Build history of the part. All positions in model axes, mm. A direction names the side the tool comes from. Coordinates: 2 decimals unless noted, no trailing zeros. Order: outer loops, then holes, each group sorted by start corner. A loop starts at its lowest first (then second) coordinate and runs counter-clockwise, first axis right, second up. Notation, with made-up numbers: M 13,-3 L 20,-3 A26 ccw 20,31 Z; hole C 15,63.5 d1. An arc over 180 degrees is marked long. Write item = value, one per line. Start each with the question number.
Q1. Pin check, flat tips, straight feed: P1, Ø3, axis at y = 0, z = 0.5, coming from the +X side; P2, Ø4, axis at y = 0, z = 0, coming from the -X side. Stop position of each tip, or through.
Q2. Drill centre lines: probe 1 along Y at (x, z) = (-0.85, 0); probe 2 along X at (y, z) = (2.25, -3). Where is each one in solid material? Low to high.
Q3. Band-saw the part on D-D on z = -4. Write the cut outline in (x, y).
Q4. Band-saw the part on C-C on x = -1.1. Write the cut outline in (y, z), plus the area to 3 significant figures.
Q5. 3-axis set-ups, long thin cutter, end or side, ignore diameter. For faces 4 (the face through (-1.51, -1.08, 4.88)), 5 (the face through (-0.5, 3.3, -0.1)): which of +Z, -Z, +X, -X, +Y, -Y reach the whole face in a straight line?
Q6. Band-saw the part on A-A on z = 0. Write the cut outline in (x, y).
Q7. Pull direction Z, two halves, no side cores. Call faces 1 (the face through (-0.3, -3, -0.1)), 2 (the face through (0, 2, 1)), 3 (the face through (-1.237, 1.617, -0.67)): released by +Z, released by -Z, zero draft, split by the parting line, or undercut.
Autodesk Inventor part; units mm, degrees
ref_plane "YZ Plane" through (0, 0, 0) normal (1, 0, 0) x (0, 1, 0)
ref_plane "XZ Plane" through (0, 0, 0) normal (0, 1, 0) x (-1, 0, 0)
ref_plane "XY Plane" through (0, 0, 0) normal (0, 0, 1) x (1, 0, 0)
sketch "Эскиз1" plane through (0, 0, 0) normal (0, 0, 1) x (1, 0, 0)
  line L0 (0, 1.75) -> (0, 3)
  line L1 (0, 3) -> (-0.5, 3)
  line L2 (-0.5, 3) -> (-0.5, 5)
  line L3 (-0.5, 5) -> (-2.5, 5)
  line L4 (-2.5, 5) -> (-2.5, 1.75)
  line L5 (-2.5, 1.75) -> (0, 1.75)
  line L6 (0, 0) -> (-4.5246, 0) construction
  dimension "d0" = 6
  dimension "d1" = 10
  dimension "d2" = 3.5
  dimension "d3" = 0.5
  dimension "d12" = 2
revolve "Вращение1" add sketch "Эскиз1" angle 360 about axis through (0, 0, 0) along (-1, 0, 0)
chamfer "Фаска1" distance 0.3 angle 45 2 edges at (-2.5, -1.75, 0) (0, -1.75, 0)
properties part number "Стопорная шайба"
Recorded:
q1.P1 = -0.05
q1.P2 = -2.45
q2.probe_1 = -5 to -1.75, 1.75 to 5
q2.probe_2 = -2.5 to -0.5
q3.outline = M -2.5,-3 L -0.5,-3 L -0.5,3 L -2.5,3 Z
q4.outline = C 0,0 d10; hole C 0,0 d3.5
q4.area = 68.9 mm2
q5.face_4 = +X, -X
q5.face_5 = +X
q6.outline = M -2.5,-5 L -0.5,-5 L -0.5,-3 L 0,-3 L 0,-2.05 L -0.3,-1.75 L -2.2,-1.75 L -2.5,-2.05 Z; M -2.5,2.05 L -2.2,1.75 L -0.3,1.75 L 0,2.05 L 0,3 L -0.5,3 L -0.5,5 L -2.5,5 Z
q7.face_1 = split by the parting line
q7.face_2 = zero draft
q7.face_3 = undercut
